Work out the finished part from the listing and answer in its coordinate system (mm). Face numbers are marked on the shaded views. Round coordinates to 2 decimals unless told otherwise and drop trailing zeros. Order: outer loops, then holes, each group sorted by start corner. A loop starts at its lowest first (then second) coordinate and runs counter-clockwise, first axis right, second up. Notation, with made-up numbers: M 8.25,-10.75 L 57.25,-10.75 A29 ccw 57.25,26.25 Z; hole C 27.5,21 d4. An arc over 180 degrees is marked long. Return JSON: item names as keys, results as strings.
from build123d import *

# Parameters (mm, degrees)
F0_W     = 22
F0_H     = 22
F1_DEPTH = 40
F2_R     = 9.169913
F3_DEPTH = 30


with BuildPart() as f1:
    # F0 (on Top) → F1 (new body)
    with BuildSketch(Plane.XY):
        with Locations((-14.504899, 3.775477)):
            Rectangle(F0_W, F0_H)
    extrude(amount=-F1_DEPTH)

    # F2 (on face) → F3 (cut)
    with BuildSketch(Plane(origin=(0, 0, -40), x_dir=(1, 0, 0), z_dir=(0, 0, -1))):
        with Locations((-14.504899, -3.775477)):
            Circle(F2_R)
    extrude(amount=-F3_DEPTH, mode=Mode.SUBTRACT)


solid = f1.part
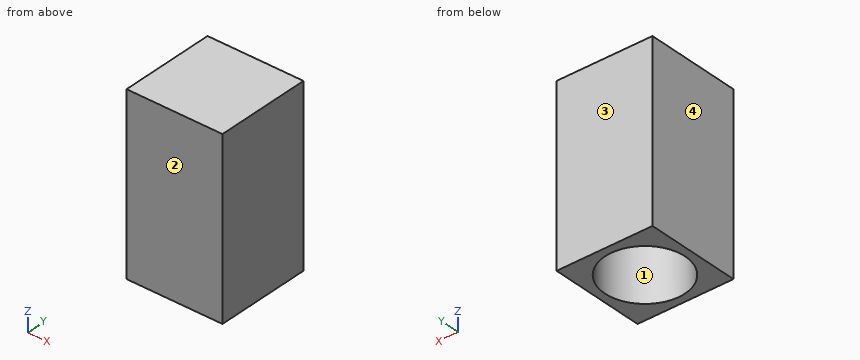
Item 1: This flat-tipped pin is pushed along its axis until it touches: pin 1 (3 mm diameter, centred on x = -15.5, y = 6, fed in from -Z). Where does it stop, or does it pass through?
Output:
{"pin 1": "stops at z = -10"}
Item 2: Find section C-C (z = -28.5). Determine the outline of the cut face in (x, y).
Output:
{"outline": "M -25.5,-7.22 L -3.5,-7.22 L -3.5,14.78 L -25.5,14.78 Z; hole C -14.5,3.78 d18.34"}
Item 3: The mould has two halves that part along Y. Classify the marked faces 1, 2, 3 and 4: pulls with the +Y half, pulls with the -Y half, needs draft (parallel to the pull), parting line crosses it, or undercut.
Output:
{"face 1": "undercut", "face 2": "pulls with the -Y half", "face 3": "pulls with the +Y half", "face 4": "needs draft"}
Item 4: Find section A-A (x = -10.25). Determine the outline of the cut face in (y, z).
Output:
{"outline": "M -7.22,-40 L -4.35,-40 L -4.35,-10 L 11.9,-10 L 11.9,-40 L 14.78,-40 L 14.78,0 L -7.22,0 Z"}
Item 5: Consider line 1 along Z through (x, y) = (-16.25, 12.25); line 2 along Y through (x, z) = (-9.5, -27.5); line 3 along Y through (x, z) = (-20.25, -25). Determine where each line is inside the solid, lowest interval first. Write a range as [from, to].
Output:
{"line 1": "z = [-10, 0]", "line 2": "y = [-7.22, -3.91], [11.46, 14.78]", "line 3": "y = [-7.22, -3.37], [10.92, 14.78]"}
Item 6: Find section B-B (y = 11.25). Determine the outline of the cut face in (x, z), plus the area to 3 significant figures.
Output:
{"outline": "M -25.5,-40 L -19.82,-40 L -19.82,-10 L -9.19,-10 L -9.19,-40 L -3.5,-40 L -3.5,0 L -25.5,0 Z", "area": "561 mm^2"}
